from build123d import *

# Parameters (mm, degrees)
F0_R     = 35
F1_DEPTH = 70
F2_T     = -5
F3_DEPTH = 20
F5_D     = 7
F5_DEPTH = 55
F5_TIP   = 2.1030121666
F6_R     = 10
F7_DEPTH = 25


with BuildPart() as f1:
    # F0 (on Top) → F1 (new body)
    with BuildSketch(Plane.XY):
        Circle(F0_R)
    extrude(amount=-F1_DEPTH)

    # F2
    f2_openings = [f1.faces().sort_by_distance(p)[0] for p in [
        (0, 0, 0),
    ]]
    offset(amount=F2_T, openings=f2_openings)

    # F3 (add): a face of the model
    f3_faces = [f1.faces().sort_by_distance(p)[0] for p in [
        (0, 0, -65),
    ]]
    extrude(f3_faces, amount=F3_DEPTH)

    # F5
    with Locations(Plane(origin=(0, 0, -70), x_dir=(1, 0, 0), z_dir=(0, 0, -1))):
        with Locations((-29, 0)):
            Hole(F5_D / 2, depth=F5_DEPTH)
            with Locations((0, 0, -(F5_DEPTH + F5_TIP / 2))):  # 118° drill point
                Cone(0, F5_D / 2, F5_TIP, mode=Mode.SUBTRACT)

    # F6 (on face) → F7 (cut, through all)
    with BuildSketch(Plane(origin=(0, 0, -70), x_dir=(1, 0, 0), z_dir=(0, 0, -1))):
        Circle(F6_R)
    extrude(amount=-F7_DEPTH, mode=Mode.SUBTRACT)


solid = f1.part
Source: CAD feature listing. Evaluate the final solid. Frame: model axes, mm. A direction names the side the tool comes from. Coordinates: 2 decimals unless noted, no trailing zeros. Loops run counter-clockwise (first coordinate to the right, second up) from the corner with the lowest first, then second, coordinate; pieces in that order, holes last. Notation, with made-up numbers: M 38,-33 L 53,-33 A22 cw 53,-11 Z; hole C 86.25,-39 d1. An arc over 180 degrees is marked long. Answer in a Markdown table with one row per item.
Q1. Set-up query: faces 4 (the conical face through (-31, 0, -14.1)), 5 (the cylindrical face through (-2.17, 9.76, -57.68)), 6 (the flat face through (0, -13, -45)). Return all of +Z, -Z, +X, -X, +Y, -Y with unobstructed straight access to the full face (end or side cutting, diameter ignored); none if empty.
Answers below:
| item | result |
|---|---|
| face 4 | -Z |
| face 5 | +Z, -Z |
| face 6 | +Z |
Q2. Section D-D on x = 19.5. Return the cut outline in (y, z).
Answers below:
| item | result |
|---|---|
| outline | M -29.06,-70 L 29.06,-70 L 29.06,0 L 22.8,0 L 22.8,-45 L -22.8,-45 L -22.8,0 L -29.06,0 Z |
Q3. Section C-C on z = -43. Return the cut outline in (x, y).
Answers below:
| item | result |
|---|---|
| outline | C 0,0 d70; hole M -29.81,-3.41 A30 ccw long -29.81,3.41 A3.5 ccw Z |
Q4. Section B-B on x = 3. Return the cut outline in (y, z), plus the area to 3 significant figures.
Answers below:
| item | result |
|---|---|
| outline | M -34.87,-70 L -9.54,-70 L -9.54,-45 L -29.85,-45 L -29.85,0 L -34.87,0 Z; M 9.54,-70 L 34.87,-70 L 34.87,0 L 29.85,0 L 29.85,-45 L 9.54,-45 Z |
| area | 1,720 mm^2 |
Q5. Ray query, probe 1 along Y at (x, z) = (0, -64); probe 2 along Y at (x, z) = (0, -24.5); probe 3 along Z at (x, y) = (21, 5.5). Return the intervals inside material, ascending. Write a range as from..to.
Answers below:
| item | result |
|---|---|
| probe 1 | y = -35..-10, 10..35 |
| probe 2 | y = -35..-30, 30..35 |
| probe 3 | z = -70..-45 |
Q6. Draft query along X for faces 1 (the cylindrical face through (27.712, -11.49, -22.185)), 2 (the flat face through (26, 16, 0)), 3 (the cylindrical face through (-28, -21, -35)). Return one class per face: pulls with the +X half, pulls with the -X half, needs draft (parallel to the pull), parting line crosses it, or undercut.
Answers below:
| item | result |
|---|---|
| face 1 | undercut |
| face 2 | needs draft |
| face 3 | parting line crosses it |
Q7. First-contact query: pin 1 (5 mm diameter, centred on y = 25.5, z = -28.5, fed in from -X); pin 2 (2 mm diameter, centred on x = -16, z = -47, fed in from +Y); pin 3 (6 mm diameter, centred on y = -25.5, z = -29.5, fed in from +X). Flat tips, straight axial feed; report the tip coordinate or a pass-through.
Answers below:
| item | result |
|---|---|
| pin 1 | stops at x = -26.38 |
| pin 2 | stops at y = 31.62 |
| pin 3 | stops at x = 26.81 |
Q8. Section A-A on y = 0. Return the cut outline in (x, z).
Answers below:
| item | result |
|---|---|
| outline | M -35,-70 L -32.5,-70 L -32.5,-15 L -30,-13.5 L -30,0 L -35,0 Z; M -25.5,-70 L -10,-70 L -10,-45 L -25.5,-45 Z; M 10,-70 L 35,-70 L 35,0 L 30,0 L 30,-45 L 10,-45 Z |
